from build123d import *

# Parameters (mm, degrees)
SKETCH1_W                       = 320
SKETCH1_H                       = 75
SKETCH1_R                       = 4.5
SKETCH1_R_2                     = 2.75
SKETCH1_R_3                     = 3.5
BOSS_EXTRUDE1_DEPTH             = 3.175
MOUNTING_AND_ACCESS_HOLES_DEPTH = 356.015056899
FILLET1_R                       = 10


with BuildPart() as part:
    # Sketch1 → Boss-Extrude1 (new body)
    with BuildSketch(Plane.XY.offset(151.125)):
        with Locations((0, 279.4)):
            Rectangle(SKETCH1_W, SKETCH1_H)
        with Locations((0, 279.4)):
            Circle(SKETCH1_R, mode=Mode.SUBTRACT)
        with Locations((27.5, 251.9)):
            Circle(SKETCH1_R_2, mode=Mode.SUBTRACT)
        with Locations((-27.5, 251.9)):
            Circle(SKETCH1_R_2, mode=Mode.SUBTRACT)
        with Locations((-27.5, 306.9)):
            Circle(SKETCH1_R_2, mode=Mode.SUBTRACT)
        with Locations((27.5, 306.9)):
            Circle(SKETCH1_R_2, mode=Mode.SUBTRACT)
        with Locations((130, 279.4)):
            Circle(SKETCH1_R_3, mode=Mode.SUBTRACT)
        with Locations((-130, 279.4)):
            Circle(SKETCH1_R_3, mode=Mode.SUBTRACT)
    extrude(amount=BOSS_EXTRUDE1_DEPTH)

    # Sketch2 → Mounting and Access Holes (cut, symmetric)
    with BuildSketch(Plane.XY.offset(154.3)):
        with BuildLine():
            Line((-124.696699141, 286.824621202), (-118.686291501, 292.835028843))
            ThreePointArc((-118.686291501, 292.835028843), (-116.564971157, 292.835028843), (-116.564971157, 290.713708499))
            Line((-116.564971157, 290.713708499), (-122.575378798, 284.703300859))
            ThreePointArc((-122.575378798, 284.703300859), (-124.696699141, 284.703300859), (-124.696699141, 286.824621202))
        make_face()
        with BuildLine():
            Line((-135.303300859, 286.824621202), (-141.313708499, 292.835028843))
            ThreePointArc((-141.313708499, 292.835028843), (-143.435028843, 292.835028843), (-143.435028843, 290.713708499))
            Line((-143.435028843, 290.713708499), (-137.424621202, 284.703300859))
            ThreePointArc((-137.424621202, 284.703300859), (-135.303300859, 284.703300859), (-135.303300859, 286.824621202))
        make_face()
        with BuildLine():
            Line((-137.424621202, 274.096699141), (-143.435028843, 268.086291501))
            ThreePointArc((-143.435028843, 268.086291501), (-143.435028843, 265.964971157), (-141.313708499, 265.964971157))
            Line((-141.313708499, 265.964971157), (-135.303300859, 271.975378798))
            ThreePointArc((-135.303300859, 271.975378798), (-135.303300859, 274.096699141), (-137.424621202, 274.096699141))
        make_face()
        with BuildLine():
            Line((-124.696699141, 271.975378798), (-118.686291501, 265.964971157))
            ThreePointArc((-118.686291501, 265.964971157), (-116.564971157, 265.964971157), (-116.564971157, 268.086291501))
            Line((-116.564971157, 268.086291501), (-122.575378798, 274.096699141))
            ThreePointArc((-122.575378798, 274.096699141), (-124.696699141, 274.096699141), (-124.696699141, 271.975378798))
        make_face()
        with BuildLine():
            Line((-50, 274.4), (-75, 274.4))
            ThreePointArc((-75, 274.4), (-80, 279.4), (-75, 284.4))
            Line((-75, 284.4), (-50, 284.4))
            ThreePointArc((-50, 284.4), (-45, 279.4), (-50, 274.4))
        make_face()
    mounting_and_access_holes = extrude(amount=MOUNTING_AND_ACCESS_HOLES_DEPTH, both=True, mode=Mode.SUBTRACT)

    # Mirror1: Mounting and Access Holes across plane
    add(mounting_and_access_holes.mirror(Plane(origin=(0, 0, 0), x_dir=(0, 0, 1), z_dir=(1, 0, 0))), mode=Mode.SUBTRACT)

    # Fillet1
    fillet1_edges = [part.edges().sort_by_distance(p)[0] for p in [
        (160, 241.9, 152.7125),
        (-160, 241.9, 152.7125),
        (-160, 316.9, 152.7125),
        (160, 316.9, 152.7125),
    ]]
    fillet(fillet1_edges, radius=FILLET1_R)


solid = part.part
Geometry: final body of the model. Coordinates: model frame, mm. Coordinates: 2 decimals unless noted, no trailing zeros. Order: outer loops, then holes, each group sorted by start corner. A loop starts at its lowest first (then second) coordinate and runs counter-clockwise, first axis right, second up.
1) Section A-A (x = -66). Return loops of the section in (y, z) (3 decimals).
Result sheet:
outline: (241.9, 151.125) - (274.4, 151.125) - (274.4, 154.3) - (241.9, 154.3) - close; (284.4, 151.125) - (316.9, 151.125) - (316.9, 154.3) - (284.4, 154.3) - close
2) Section C-C (x = 130). Return loops of the section in (y, z) (3 decimals).
Result sheet:
outline: (241.9, 151.125) - (275.9, 151.125) - (275.9, 154.3) - (241.9, 154.3) - close; (282.9, 151.125) - (316.9, 151.125) - (316.9, 154.3) - (282.9, 154.3) - close
3) First-contact query: P1, Ø3.5, axis at x = 27.5, y = 306.9, coming from the +Z side. Flat tip, straight axial feed; report the tip coordinate or a pass-through.
Result sheet:
P1: passes through
4) Draft query along Y for faces 1 (the flat face through (-2, 272, 151.125)), 2 (the cylindrical face through (-157.15, 244.91, 152.73)), 3 (the cylindrical face through (-28.096, 304.215, 152.69)), 4 (the flat face through (-140.47, 287.75, 152.69)). Return one class per face: released by +Y, released by -Y, zero draft, split by the parting line, or undercut.
Result sheet:
face 1: zero draft
face 2: released by -Y
face 3: undercut
face 4: undercut
5) Section B-B (x = 27.5). Return loops of the section in (y, z) (3 decimals).
Result sheet:
outline: (241.9, 151.125) - (249.15, 151.125) - (249.15, 154.3) - (241.9, 154.3) - close; (254.65, 151.125) - (304.15, 151.125) - (304.15, 154.3) - (254.65, 154.3) - close; (309.65, 151.125) - (316.9, 151.125) - (316.9, 154.3) - (309.65, 154.3) - close
6) Ray query, probe 1 along Y at (x, z) = (27.5, 153.2); probe 2 along X at (y, z) = (266, 153.8); probe 3 along X at (y, z) = (279.4, 153.05). Return the intervals inside material, ascending.
Result sheet:
probe 1: y = 241.9 to 249.15, 254.65 to 304.15, 309.65 to 316.9
probe 2: x = -160 to -143.47, -141.28 to -118.72, -116.53 to 116.53, 118.72 to 141.28, 143.47 to 160
probe 3: x = -160 to -133.5, -126.5 to -80, -45 to -4.5, 4.5 to 45, 80 to 126.5, 133.5 to 160
